Read the model definition and answer for the solid it produces. Units are mm, in the model's axes. Coordinates: 2 decimals unless noted, no trailing zeros. Loops run counter-clockwise (first coordinate to the right, second up) from the corner with the lowest first, then second, coordinate; pieces in that order, holes last. Notation, with made-up numbers: (-14.75, 2.25) -> (13.25, 2.25) arc R12 ccw to (13.25, 23.25) -> close; hole circle Ø5 at (-16.5, 79). An arc over 180 degrees is marked (long way). Answer as a JSON object with one key per item and string values. Group by question number.
Q1. The part is cut by section D-D on z = -56. Write down the section's boundary in (x, y), and give its area (3 significant figures).
Q2. Straight lines are drawn through the part: line 1 along X through (y, z) = (5, -16.5); line 2 along Z through (x, y) = (27.5, 6.75); line 3 along X through (y, z) = (2.75, 7). For each, find the intervals that lie inside material, in ascending order. Write a range as [from, to].
Q3. The part is cut by section A-A on z = -12.7. Write down the section's boundary in (x, y).
Q4. The part is cut by section C-C on x = -57.5. Write down the section's boundary in (y, z).
Q5. Each of these flat-tipped pins is pushed along its axis until it touches: P1, Ø3, axis at y = 4, z = 14.5, coming from the -X side; P2, Ø3, axis at x = -35.23, z = -16.46, coming from the +Y side; P3, Ø1.5, axis at x = -53.5, y = 3, coming from the -Z side. Where does it stop, or does it pass through?
Q6. The part is cut by section B-B on y = 4.75. State how many separate pieces and enclosed holes the cut face has, and give its area (3 significant figures).
Autodesk Inventor part; units mm, degrees
ref_plane "YZ Plane" through (0, 0, 0) normal (1, 0, 0) x (0, 1, 0)
ref_plane "XZ Plane" through (0, 0, 0) normal (0, 1, 0) x (-1, 0, 0)
ref_plane "XY Plane" through (0, 0, 0) normal (0, 0, 1) x (1, 0, 0)
sketch "Sketch1" plane through (0, 0, 0) normal (0, 1, 0) x (-1, 0, 0)
  line L0 (0, 0) -> (67.2338, 0)
  arc A0 (76.7588, -9.525) -> (67.2338, 0) centre (67.2338, -9.525) ccw
  arc A1 (67.2338, -48.9204) -> (76.7588, -39.3954) centre (67.2338, -39.3954) ccw
  line L1 (76.7588, -9.525) -> (76.7588, -39.3954)
  line L2 (67.2338, -48.9204) -> (15.367, -48.9204)
  line L3 (15.367, -48.9204) -> (-3.6891, -67.9765)
  line L4 (0, 0) -> (-25.3962, 25.3962)
  circle A2 centre (35.2298, -16.4592) radius 1.905
  circle A3 centre (35.2298, -32.4612) radius 1.905
  circle A4 centre (67.2338, -32.4612) radius 1.905
  circle A5 centre (67.2338, -16.4592) radius 1.905
  circle A6 centre (-26.1112, -24.4602) radius 1.85
  circle A7 centre (-26.1112, 7.2898) radius 1.85
  line L5 (-25.3962, 25.3962) -> (-31.7462, 25.3962)
  line L6 (-31.7462, 25.3962) -> (-31.7462, -39.9194)
  line L7 (-31.7462, -39.9194) -> (-3.6891, -67.9765)
  circle A8 centre (0, -12.7) radius 1.85
  circle A9 centre (0, -38.1) radius 1.85
  line L8 (-3.6891, -67.9765) -> (-12.6694, -58.9962)
  circle A10 centre (-3.6891, -59.4929) radius 1.85
  circle A11 centre (-17.1882, -44.4383) radius 1.85
  dimension "d21" = 6.35
extrude "Extrusion1" add sketch "Sketch1" along normal blind 7
properties part number "MotorSuspension"
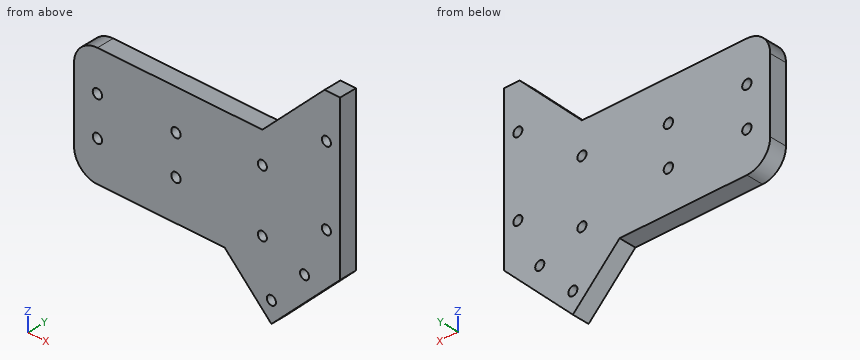
Final values:
{
 "1": {"outline": "(-8.29, 0) -> (15.67, 0) -> (15.67, 7) -> (-8.29, 7) -> close", "area": "168 mm2"},
 "2": {"line 1": "x = [-76.76, -69.14], [-65.33, -37.13], [-33.33, 31.75]", "line 2": "z = [-44.17, -25.68], [-23.24, 6.07], [8.51, 25.4]", "line 3": "x = [7, 24.28], [27.94, 31.75]"},
 "3": {"outline": "(-76.76, 0) -> (-1.85, 0) -> (-1.85, 7) -> (-76.76, 7) -> close; (1.85, 0) -> (31.75, 0) -> (31.75, 7) -> (1.85, 7) -> close"},
 "4": {"outline": "(0, -48.92) -> (7, -48.92) -> (7, 0) -> (0, 0) -> close"},
 "5": {"P1": "stops at x = 13", "P2": "passes through", "P3": "stops at z = -48.92"},
 "6": {"separate pieces": "1", "enclosed holes": "10", "area": "5,970 mm2"}
}
